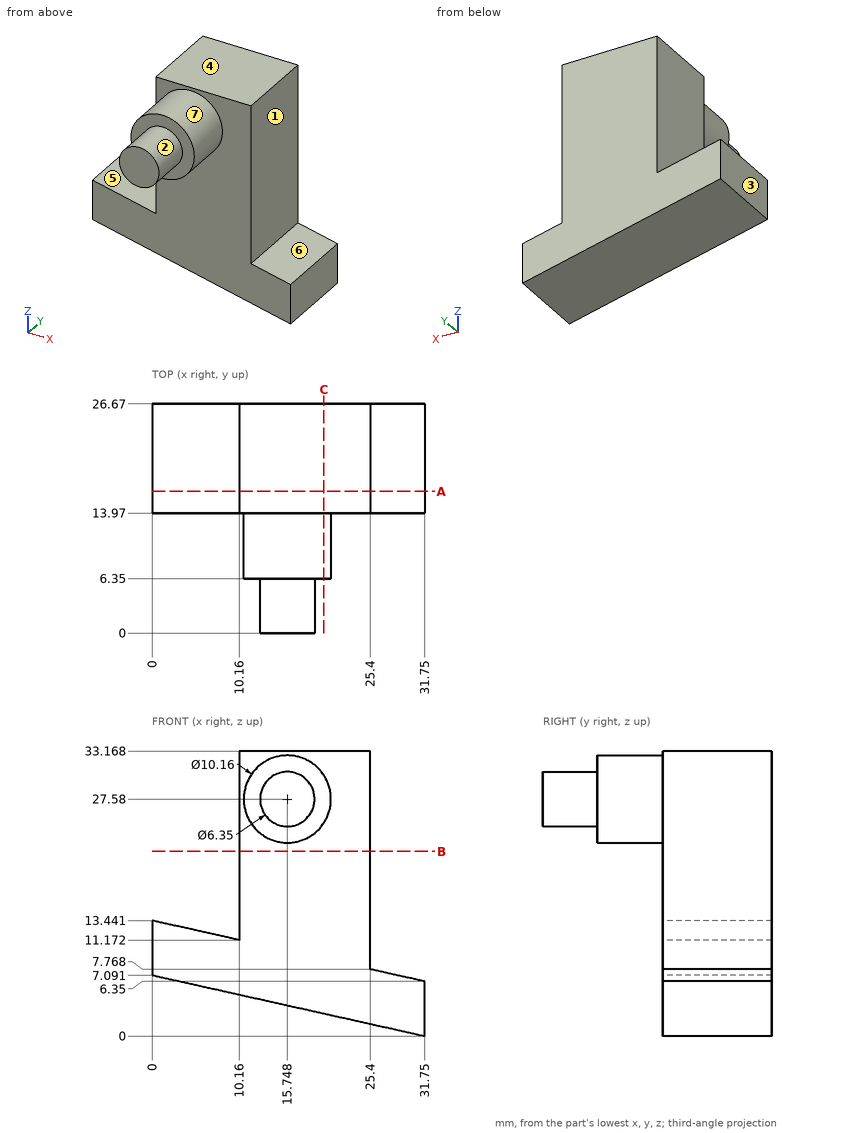
Can you work these out from the drawing? Everything is in mm from the part's minimum corner. A direction names the side the tool comes from. Round coordinates to 2 decimals unless told otherwise and drop trailing zeros. Loops run counter-clockwise (first coordinate to the right, second up) from the corner with the lowest first, then second, coordinate; pieces in that order, holes last. Notation, with made-up numbers: M -23,8.25 L 31,8.25 A18 ccw 31,36.25 Z; hole C -22.75,54.25 d5. An arc over 180 degrees is marked long. Write item = value, one per line.
1. I want a section at C-C, the plane x = 20. Write out the boundary of the cut face in (y, z).
Results below:
outline = M 6.35,24.8 L 13.97,24.8 L 13.97,2.62 L 26.67,2.62 L 26.67,33.17 L 13.97,33.17 L 13.97,30.36 L 6.35,30.36 Z
2. Will these pins go through, and if not, where does the flat tip stop? P1, Ø5, axis at y = 13, z = 18, coming from the -X side; P2, Ø3, axis at x = 14, z = 6, coming from the -Y side; P3, Ø10, axis at y = 19.5, z = 26.5, coming from the +X side.
Results below:
P1 = 10.16
P2 = 13.97
P3 = 25.4
3. Which directions (+Z, -Z, +X, -X, +Y, -Y) give clear straight access to the entire face, cutting with the end or side of a thin tool? Please do the marked faces 1, 2 and 3.
Results below:
face_1 = +Z, +X, +Y, -Y
face_2 = -Y
face_3 = +Z, -Z, -X, +Y, -Y
4. I need wall thicknesses on probe 1 along Y at (x, z) = (7.5, 7); probe 2 along X at (y, z) = (21.25, 24); probe 3 along Y at (x, z) = (11, 29). Which ranges of each line are inside material? Lowest first, please.
Results below:
probe_1 = 13.97 to 26.67
probe_2 = 10.16 to 25.4
probe_3 = 6.35 to 26.67
5. I want a section at A-A, the plane y = 16.5. Write out the boundary of the cut face in (x, z), and give its area (3 significant figures).
Results below:
outline = M 0,7.09 L 31.75,0 L 31.75,6.35 L 25.4,7.77 L 25.4,33.17 L 10.16,33.17 L 10.16,11.17 L 0,13.44 Z
area = 563 mm²
6. I want a section at B-B, the plane z = 21.5. Write out the boundary of the cut face in (x, y), and give its area (3 significant figures).
Results below:
outline = M 10.16,13.97 L 25.4,13.97 L 25.4,26.67 L 10.16,26.67 Z
area = 194 mm²
7. Thinking about a two-plate mould opening in X: for the marked faces 4, 5, 6 and 7, which applies, +X half, -X half, draft (parallel to the pull), parting line (faces both ways), or undercut?
Results below:
face_4 = draft
face_5 = undercut
face_6 = +X half
face_7 = parting line
